The model under review builds one solid part; all positions refer to its coordinate system, in mm. Face numbers are marked on the shaded views. A direction names the side the tool comes from. Give positions to 0.01 mm unless a question says otherwise; leave off trailing zeros. Write each loop counter-clockwise with the first axis right and the second up, starting at its lowest first coordinate (ties: lowest second). Pieces come first, ordered by that corner, then holes. Notation, with made-up numbers: (26.5, -35.5) -> (36.5, -35.5) arc R28 cw to (36.5, -15.5) -> close; hole circle Ø4 at (22, 53.25). An arc over 180 degrees is marked (long way). Use CSV: the item, a comma, the result in double quotes.
```python
from build123d import *

# Parameters (mm, degrees)
SKETCH_R        = 32
PAD_DEPTH       = 15
PAD001_DEPTH    = 5
SKETCH002_R     = 19
PAD002_DEPTH    = 15
SKETCH003_R     = 27.5
SKETCH003_R_2   = 21.5
POCKET_DEPTH    = 5
SKETCH004_R     = 21.5
PAD003_DEPTH    = 15
SKETCH005_R     = 17
POCKET001_DEPTH = 45.001
SKETCH006_R     = 10
POCKET002_DEPTH = 30.001


with BuildPart() as part:
    # Sketch → Pad (new body, symmetric)
    with BuildSketch(Plane.XZ):
        Circle(SKETCH_R)
    extrude(amount=PAD_DEPTH, both=True)

    # Sketch001 → Pad001 (join, symmetric)
    with BuildSketch(Plane.XZ):
        with BuildLine():
            ThreePointArc((26.6782831974, 17.6711404736), (-1.75595e-05, 32), (-26.678302591, 17.671111195))
            ThreePointArc((-26.678302591, 17.671111195), (-16.8367727335, 42.9140409584), (-18.3212438006, 69.9669069549))
            ThreePointArc((-18.3212438006, 69.9669069549), (-1.6382e-05, 56), (18.3212351214, 69.9668753614))
            ThreePointArc((18.3212351214, 69.9668753614), (16.8367725476, 42.9140421212), (26.6782831975, 17.6711404736))
        make_face()
    extrude(amount=PAD001_DEPTH, both=True)

    # Sketch002 → Pad002 (join, symmetric)
    with BuildSketch(Plane.XZ):
        with Locations((0, 75)):
            Circle(SKETCH002_R)
    extrude(amount=PAD002_DEPTH, both=True)

    # Sketch003 (on Face10 of Pad002) → Pocket (cut)
    with BuildSketch(Plane.XZ.offset(15)):
        Circle(SKETCH003_R)
        Circle(SKETCH003_R_2, mode=Mode.SUBTRACT)
    extrude(amount=-POCKET_DEPTH, mode=Mode.SUBTRACT)

    # Sketch004 (on Face14 of Pocket) → Pad003 (join)
    with BuildSketch(Plane.XZ.offset(15)):
        Circle(SKETCH004_R)
    extrude(amount=PAD003_DEPTH)

    # Sketch005 (on Face15 of Pad003) → Pocket001 (cut, through all)
    with BuildSketch(Plane.XZ.offset(30)):
        Circle(SKETCH005_R)
    extrude(amount=-POCKET001_DEPTH, mode=Mode.SUBTRACT)

    # Sketch006 (on Face3 of Pocket001) → Pocket002 (cut, through all)
    with BuildSketch(Plane.XZ.offset(15)):
        with Locations((0, 75)):
            Circle(SKETCH006_R)
    extrude(amount=-POCKET002_DEPTH, mode=Mode.SUBTRACT)


solid = part.part
```
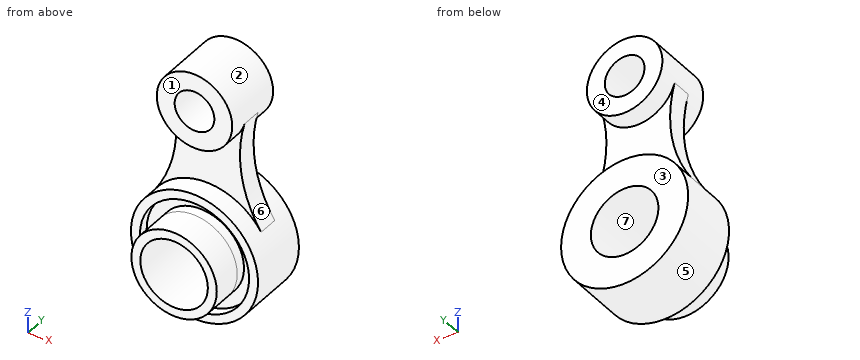
Q1. Consider section D-D (x = 12.5). Write out the cut boundary in (y, z), then the cut area to 3 significant figures.
Derived:
outline,"(-30, -17.49) -> (-10, -17.49) -> (-10, -24.49) -> (-15, -24.49) -> (-15, -29.46) -> (15, -29.46) -> (15, -11.52) -> (-30, -11.52) -> close; (-30, 11.52) -> (15, 11.52) -> (15, 29.46) -> (5, 29.46) -> (5, 60.69) -> (15, 60.69) -> (15, 89.31) -> (-15, 89.31) -> (-15, 60.69) -> (-5, 60.69) -> (-5, 29.46) -> (-15, 29.46) -> (-15, 24.49) -> (-10, 24.49) -> (-10, 17.49) -> (-30, 17.49) -> close"
area,"2,360 mm2"
Q2. The part is to be moulded in two halves that separate along X. For the marked faces 4, 5, 6 and 7, say which applies: pulls with the +X half, pulls with the -X half, needs draft (parallel to the pull), parting line crosses it, or undercut.
Derived:
face 4,"needs draft"
face 5,"parting line crosses it"
face 6,"pulls with the +X half"
face 7,"undercut"
Q3. To check wall thickness, follow probe 1 along Z at (x, y) = (0, -11.25); probe 2 along Z at (x, y) = (0, -4); probe 3 along Y at (x, z) = (25.5, -11). State the ranges of each line that lie inside material, in increasing order.
Derived:
probe 1,"z = -32 to -27.5, -21.5 to -17, 17 to 21.5, 27.5 to 32, 56 to 65, 85 to 94"
probe 2,"z = -32 to -17, 17 to 65, 85 to 94"
probe 3,"y = -15 to 15"
Q4. Consider section A-A (x = 0). Write out the cut boundary in (y, z).
Derived:
outline,"(-30, -21.5) -> (-10, -21.5) -> (-10, -27.5) -> (-15, -27.5) -> (-15, -32) -> (15, -32) -> (15, -17) -> (-30, -17) -> close; (-30, 17) -> (15, 17) -> (15, 32) -> (5, 32) -> (5, 56) -> (15, 56) -> (15, 65) -> (-15, 65) -> (-15, 56) -> (-5, 56) -> (-5, 32) -> (-15, 32) -> (-15, 27.5) -> (-10, 27.5) -> (-10, 21.5) -> (-30, 21.5) -> close; (-15, 85) -> (15, 85) -> (15, 94) -> (-15, 94) -> close"
Q5. Consider section C-C (z = 0). Write out the cut boundary in (x, y).
Derived:
outline,"(-32, -15) -> (-27.5, -15) -> (-27.5, -10) -> (-21.5, -10) -> (-21.5, -30) -> (-17, -30) -> (-17, 15) -> (-32, 15) -> close; (17, -30) -> (21.5, -30) -> (21.5, -10) -> (27.5, -10) -> (27.5, -15) -> (32, -15) -> (32, 15) -> (17, 15) -> close"
Q6. Consider section B-B (z = 75). Write out the cut boundary in (x, y).
Derived:
outline,"(-19, -15) -> (-10, -15) -> (-10, 15) -> (-19, 15) -> close; (10, -15) -> (19, -15) -> (19, 15) -> (10, 15) -> close"
Q7. Machinability: for the marked faces 1, 2 and 3, which of the approach directions +Z, -Z, +X, -X, +Y, -Y give a long, thin tool a straight path to every point of the face, cutting with its end or side? Answer none if there is none.
Derived:
face 1,"+Z, +X, -X, -Y"
face 2,"none"
face 3,"+Z, -Z, +X, -X, +Y"
Q8. Insertion check: pin 1 (4 mm diameter, centred on y = 7.5, z = -10, fed in from -X); pin 2 (6 mm diameter, centred on x = 14, y = -21.5, fed in from +Z); pin 3 (5 mm diameter, centred on x = 13, z = 2, fed in from +Y) (3 decimals); pin 4 (1 mm diameter, centred on x = -21.5, y = 9.5, fed in from -Z). Each pin has a flat end and moves straight along its axis. Give the tip position at first contact, or say it passes through.
Derived:
pin 1,"stops at x = -30.98"
pin 2,"stops at z = 18.47"
pin 3,"passes through"
pin 4,"stops at z = -24.15"
